from build123d import *

# Parameters (mm, degrees)
BOSS_EXTRUDE1_DEPTH                             = 25.4
CBORE_FOR_10_SOCKET_HEAD_CAP_SCREW1_D           = 5.1054
CBORE_FOR_10_SOCKET_HEAD_CAP_SCREW1_CBORE_D     = 9.144
CBORE_FOR_10_SOCKET_HEAD_CAP_SCREW1_CBORE_DEPTH = 4.826
M3X0_5_TAPPED_HOLE1_D                           = 2.5
FILLET1_R                                       = 2.54


with BuildPart() as part:
    # Sketch1 → Boss-Extrude1 (new body)
    with BuildSketch(Plane(origin=(0, 0, 0), x_dir=(1, 0, 0), z_dir=(0, 1, 0))):
        Polygon((0, 0), (22.225, 0), (22.225, 9.525), (-6.35, 9.525), (-9.525, -11.1125), (-9.525, -17.4625), (-6.35, -28.575), (0, -28.575), align=None)
    extrude(amount=BOSS_EXTRUDE1_DEPTH)

    # CBORE for #10 Socket Head Cap Screw1 (through all)
    with Locations(Plane.XY):
        with Locations((6.35, 17.4625), (15.875, 7.9375), (6.35, 7.9375), (15.875, 17.4625)):
            CounterBoreHole(CBORE_FOR_10_SOCKET_HEAD_CAP_SCREW1_D / 2, CBORE_FOR_10_SOCKET_HEAD_CAP_SCREW1_CBORE_D / 2, CBORE_FOR_10_SOCKET_HEAD_CAP_SCREW1_CBORE_DEPTH)

    # M3x0.5 Tapped Hole1 (through all)
    with Locations(Plane(origin=(0, 0, 0), x_dir=(0, 0, -1), z_dir=(1, 0, 0))):
        with Locations((-14.2875, 16.7), (-14.2875, 8.7)):
            Hole(M3X0_5_TAPPED_HOLE1_D / 2)

    # Fillet1
    fillet1_edges = [part.edges().sort_by_distance(p)[0] for p in [
        (22.225, 0, -4.7625),
        (22.225, 25.4, -4.7625),
        (-3.175, 25.4, 28.575),
        (-3.175, 0, 28.575),
    ]]
    fillet(fillet1_edges, radius=FILLET1_R)


solid = part.part
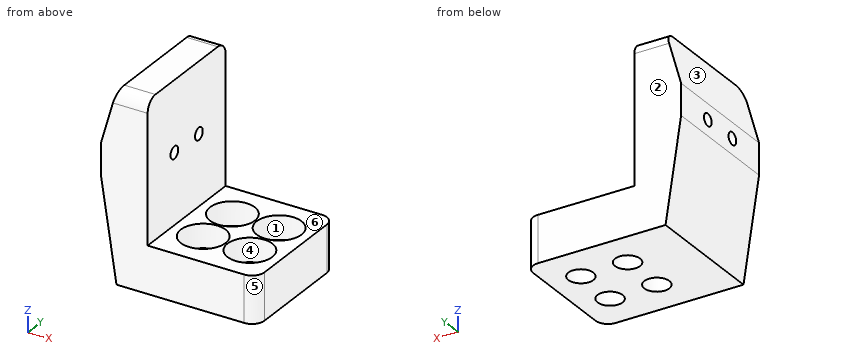
Model file for the job. Use its own axes, mm. Face numbers are marked on the shaded views. A direction names the side the tool comes from. Give positions to 0.01 mm unless a question says otherwise; leave off trailing zeros.
Item 1: Drop flat-ended pins along their axis: P1, Ø10, axis at x = 8, y = 19.5, coming from the +Z side; P2, Ø4.5, axis at x = 5, y = 9, coming from the +Z side; P3, Ø1, axis at y = 10.5, z = 9, coming from the -X side. Give the stop position or say it passes through.
Check values:
P1: stops at z = 0
P2: stops at z = -4.83
P3: stops at x = -9.28
Item 2: Drill centre lines: line 1 along Y through (x, z) = (6.35, -7.9); line 2 along Y through (x, z) = (6, -2); line 3 along Z through (x, y) = (4.5, 13.5) (3 decimals). Where is each one in solid material? Low to high.
Check values:
line 1: y = 0 to 5.38, 10.49 to 14.91, 20.02 to 25.4
line 2: y = 0 to 3.38, 12.5 to 12.9, 22.02 to 25.4
line 3: z = -9.525 to -4.826
Item 3: Which spindle directions (+Z, -Z, +X, -X, +Y, -Y) get a long thin tool onto all of the face, cutting with end or side? Do the marked faces 4, 5 and 6. Say none if no direction does.
Check values:
face 4: +Z
face 5: +Z, -Z, +X, -Y
face 6: +Z, +X, +Y, -Y
Item 4: Mould opens along X. For the marked faces 1, 2 and 3 say: +X half, -X half, draft (parallel to the pull), parting line (faces both ways), or undercut.
Check values:
face 1: undercut
face 2: draft
face 3: -X half
Item 5: Slice it at A-A (x = 6.35). Give the number of separate pieces and of enclosed holes in the cut face, plus the area to 3 significant figures.
Check values:
separate pieces: 3
enclosed holes: 0
area: 106 mm2
